Autodesk Inventor part; units mm, degrees
ref_plane "YZ Plane" through (0, 0, 0) normal (1, 0, 0) x (0, 1, 0)
ref_plane "XZ Plane" through (0, 0, 0) normal (0, 1, 0) x (-1, 0, 0)
ref_plane "XY Plane" through (0, 0, 0) normal (0, 0, 1) x (1, 0, 0)
sketch "Sketch1" plane through (0, 0, 0) normal (0, 1, 0) x (-1, 0, 0)
  line L0 (0, 0) -> (0, -62.5)
  line L1 (9.458, 0) -> (9.458, 12.5)
  line L2 (9.458, 12.5) -> (9.458, -12.5)
  line L3 (9.458, 12.5) -> (-14.404, 12.5)
  line L4 (-14.404, 12.5) -> (-14.404, -12.5)
  line L5 (-14.404, -12.5) -> (9.458, -12.5)
  line L6 (-14.404, 12.5) -> (-12.404, 12.5)
  line L7 (-14.404, -12.5) -> (-12.404, -12.5)
  circle A0 centre (0.096, 10.5) radius 1.1
  circle A1 centre (-12.404, 10.5) radius 1.1
  circle A2 centre (-12.404, -10.5) radius 1.1
  circle A3 centre (0.096, -10.5) radius 1.1
  line L8 (9.458, -62.5) -> (9.458, -50)
  line L9 (9.458, -50) -> (9.458, -75)
  line L10 (9.458, -50) -> (-14.404, -50)
  line L11 (-14.404, -50) -> (-14.404, -75)
  line L12 (-14.404, -75) -> (9.458, -75)
  line L13 (-14.404, -50) -> (-12.404, -50)
  line L14 (-14.404, -75) -> (-12.404, -75)
  circle A4 centre (0.096, -52) radius 1.1
  circle A5 centre (-12.404, -52) radius 1.1
  circle A6 centre (-12.404, -73) radius 1.1
  circle A7 centre (0.096, -73) radius 1.1
  line L15 (12.458, 15.5) -> (-17.404, 15.5)
  line L16 (-17.404, 15.5) -> (-17.404, -78)
  line L17 (-17.404, -78) -> (12.458, -78)
  line L18 (12.458, -78) -> (12.458, 15.5)
  line L19 (-14.404, -12.5) -> (-14.404, -50)
  line L20 (9.458, -50) -> (9.458, -12.5)
extrude "Extrusion1" add sketch "Sketch1" against normal blind 3 contours L5 L4 L3 L1 L2 | L5 L20 L10 L0 | L0 L10 L19 L5 | L10 L8 L9 L12 L11 | L18 L17 L16 L15
sketch "Sketch2" plane through (0, 0, 0) normal (0, 1, 0) x (1, 0, 0)
  circle A0 centre (-0.096, -10.5) radius 1.1
  circle A1 centre (-0.096, -10.5) radius 2
  circle A2 centre (12.404, -10.5) radius 1.1
  circle A3 centre (12.404, -10.5) radius 2
  circle A4 centre (12.404, 10.5) radius 1.1
  circle A5 centre (12.404, 10.5) radius 2
  circle A6 centre (-0.096, 10.5) radius 2
  circle A7 centre (-0.096, 52) radius 1.1
  circle A8 centre (-0.096, 52) radius 2
  circle A9 centre (-0.096, 73) radius 1.1
  circle A10 centre (-0.096, 73) radius 2
  circle A11 centre (12.404, 73) radius 1.1
  circle A12 centre (12.404, 73) radius 2
  circle A13 centre (12.404, 52) radius 1.1
  circle A14 centre (12.404, 52) radius 2
  circle A15 centre (-0.096, 73) radius 1.1
  circle A16 centre (12.404, 73) radius 1.1
  circle A17 centre (12.404, 52) radius 1.1
  circle A18 centre (-0.096, 52) radius 1.1
  circle A19 centre (-0.096, 10.5) radius 1.1
  circle A20 centre (12.404, 10.5) radius 1.1
  circle A21 centre (12.404, -10.5) radius 1.1
  circle A22 centre (-0.096, -10.5) radius 1.1
  circle A23 centre (-0.096, 10.5) radius 1.1
  point P0 (0, 0)
  dimension "d21" = 4
  dimension "d22" = 4
  dimension "d23" = 4
  dimension "d24" = 4
  dimension "d25" = 4
  dimension "d26" = 4
  dimension "d27" = 4
  dimension "d28" = 4
extrude "Extrusion2" add sketch "Sketch2" along normal blind 3
extrude "Extrusion3" add sketch "Sketch1" along normal blind 4 contours L18 L17 L16 L15
sketch "Sketch3" plane through (-12.458, -3, -78) normal (-1, 0, 0) x (0, 0, 1)
  line L0 (89.6, 0) -> (87.4, 0)
  line L1 (68.6, 0) -> (66.4, 0)
  line L2 (27.1, 0) -> (24.9, 0)
  line L3 (6.1, 0) -> (3.9, 0)
  line L4 (88.5, 0) -> (88.5, 3)
  line L5 (88.5, 3) -> (88.5, 5)
  line L6 (88.5, 3) -> (88.5, 6)
  line L7 (88.5, 5) -> (67.5, 5)
  line L8 (67.5, 3) -> (67.5, 6)
  line L9 (67.5, 5) -> (67.5, 3)
  line L10 (67.5, 3) -> (88.5, 3)
  line L11 (27.1, 0) -> (24.9, 0)
  line L12 (26, 0) -> (26, 5)
  line L13 (26, 5) -> (5, 5)
  line L14 (5, 3) -> (5, 6)
  line L15 (5, 5) -> (5, 3)
  line L16 (26, 3) -> (5, 3)
  line L17 (5, 3) -> (26, 3)
  dimension "d33" = 2
  dimension "d34" = 5
extrude "Extrusion4" cut sketch "Sketch3" against normal up to surface (3 mm away)
sketch "Sketch4" plane through (-12.458, -3, -78) normal (-1, 0, 0) x (0, 0, 1)
  line L0 (0, 0) -> (93.5, 0)
  line L1 (78, 0) -> (78, -30)
  line L2 (78, -30) -> (83, -30)
  line L3 (83, -30) -> (73, -30)
  line L4 (73, -30) -> (73, 0)
  line L5 (83, -30) -> (83, 0)
  line L6 (73, 0) -> (83, 0)
  line L7 (78, 3) -> (78, -30)
  point P0 (78, -30)
  point P1 (83, 0)
  point P2 (73, 0)
  dimension "d37" = 30
  dimension "d38" = 5
  dimension "d39" = 10
extrude "Extrusion5" add sketch "Sketch4" against normal up to surface (29.862 mm away)
sketch "Sketch5" plane through (-12.458, -33, 5) normal (0, 0, 1) x (1, 0, 0)
  line L0 (0, 0) -> (29.862, 0)
  line L1 (0, 30) -> (0, 0)
  circle A0 centre (14.931, 15) radius 15
  line L2 (29.862, 30) -> (29.862, 0)
  line L3 (29.862, 0) -> (29.862, 15)
  point P0 (12.458, 33)
  point P1 (29.862, 13.5629)
  point P2 (14.931, 0)
  point P3 (0, 13.5629)
extrude "Extrusion6" cut sketch "Sketch5" against normal up to surface (10 mm away) contours L1 A0 L0 | A0 L2 L0
sketch "Sketch6" plane through (-12.458, -3, 5) normal (0, 0, 1) x (1, 0, 0)
  line L0 (29.862, -30) -> (29.862, 0)
  line L1 (29.862, -16.4371) -> (26.862, -16.4371)
  circle A0 centre (26.862, -16.4371) radius 1.1
  arc A1 (0, -16.4371) -> (29.862, -16.4371) centre (14.931, -15) ccw
  circle A2 centre (14.931, -15) radius 4.093
  circle A3 centre (25.9738, -19.7402) radius 1.1
  circle A4 centre (24.191, -22.6593) radius 1.1
  circle A5 centre (21.6581, -24.9579) radius 1.1
  circle A6 centre (18.5801, -26.4498) radius 1.1
  circle A7 centre (15.2065, -27.0141) radius 1.1
  circle A8 centre (11.8106, -26.605) radius 1.1
  circle A9 centre (8.6675, -25.2558) radius 1.1
  circle A10 centre (6.0318, -23.0758) radius 1.1
  circle A11 centre (4.1171, -20.2414) radius 1.1
  circle A12 centre (3.0784, -16.9825) radius 1.1
  circle A13 centre (3, -13.5629) radius 1.1
  point P0 (12.458, 3)
  dimension "d46" = 3
  dimension "d47" = 2.2
  dimension "d50" = 180
extrude "Extrusion7" cut sketch "Sketch6" against normal up to surface (10 mm away) contours A0 | A3 | A4 | A5 | A6 | A7 | A8 | A9 | A10 | A11 | A12 | A13
sketch "Sketch7" plane through (-12.458, -3, 5) normal (0, 0, 1) x (1, 0, 0)
  arc A0 (0, -16.4371) -> (29.862, -16.4371) centre (14.931, -15) ccw
  circle A1 centre (14.931, -15) radius 2
  point P0 (12.458, 3)
  dimension "d54" = 4
extrude "Extrusion8" cut sketch "Sketch7" against normal up to surface (10 mm away)
sketch "Sketch8" plane through (0, 4, 0) normal (0, 1, 0) x (1, 0, 0)
  line L0 (17.404, -15.5) -> (17.404, 78)
  line L1 (17.404, 78) -> (-12.458, 78)
  line L2 (-12.458, 78) -> (-12.458, -15.5)
  line L3 (-12.458, -15.5) -> (17.404, -15.5)
  line L4 (14.404, 75) -> (14.404, -12.5)
  line L5 (14.404, -12.5) -> (-9.458, -12.5)
  line L6 (-9.458, -12.5) -> (-9.458, 75)
  line L7 (-9.458, 75) -> (14.404, 75)
  line L8 (-9.458, -13) -> (14.404, -13)
  line L9 (14.404, -13) -> (14.904, -13)
  line L10 (14.904, -13) -> (14.904, 75)
  line L11 (14.904, 75) -> (14.904, 75.5)
  line L12 (14.904, 75.5) -> (-9.458, 75.5)
  line L13 (-9.458, 75.5) -> (-9.958, 75.5)
  line L14 (-9.958, 75.5) -> (-9.958, -13)
  line L15 (-12.458, 78) -> (-12.458, -15.5)
  line L16 (-9.958, -13) -> (-9.458, -13)
  point P0 (0, 0)
  dimension "d57" = 0.5
  dimension "d58" = 0.5
  dimension "d59" = 0.5
  dimension "d60" = 0.5
extrude "Extrusion9" cut sketch "Sketch8" against normal up to surface (4 mm away) contours L16 L14 L13 L12 L11 L10 L9 L8
sketch "Sketch9" plane through (0, -3, 0) normal (0, -1, 0) x (1, 0, 0)
  circle A0 centre (12.404, -31.25) radius 1.45
  circle A1 centre (-0.096, -31.25) radius 1.45
  arc A2 (14.904, -29.5917) -> (14.904, -32.9083) centre (12.404, -31.25) ccw
  circle A3 centre (-0.096, -31.25) radius 3
  point P0 (0, 0)
extrude "Extrusion10" cut sketch "Sketch9" against normal up to surface (7 mm away) contours A0 | A1
sketch "Sketch10" plane through (0, -3, 0) normal (0, -1, 0) x (1, 0, 0)
  circle A0 centre (12.404, 10.5) radius 1.1
  circle A1 centre (-0.096, 10.5) radius 1.1
  circle A2 centre (12.404, -10.5) radius 1.1
  circle A3 centre (-0.096, -10.5) radius 1.1
  circle A4 centre (-0.096, -52) radius 1.1
  circle A5 centre (12.404, -52) radius 1.1
  circle A6 centre (12.404, -73) radius 1.1
  circle A7 centre (-0.096, -73) radius 1.1
  point P0 (0, 0)
extrude "Extrusion11" add sketch "Sketch10" against normal blind 3
sketch "Sketch11" plane through (0, -3, 0) normal (0, -1, 0) x (1, 0, 0)
  line L0 (17.404, -78) -> (-12.458, -78)
  line L1 (-12.458, -78) -> (-12.458, -85)
  line L2 (-12.458, -85) -> (17.404, -85)
  line L3 (17.404, -85) -> (17.404, -78)
  circle A0 centre (12.404, -81.5) radius 1.45
  circle A1 centre (0, -81.5) radius 1.45
  line L4 (-12.458, 15.5) -> (17.404, 15.5)
  line L5 (-12.458, 15.5) -> (-12.458, 22.5)
  line L6 (-12.458, 22.5) -> (17.404, 22.5)
  line L7 (17.404, 22.5) -> (17.404, 15.5)
  line L8 (17.404, 15.5) -> (-12.458, 15.5)
  line L9 (-12.458, -78) -> (17.404, -78)
  circle A2 centre (12.404, 19) radius 1.45
  circle A3 centre (0, 19) radius 1.45
  point P0 (0, 0)
  dimension "d67" = 7
  dimension "d69" = 2.9
  dimension "d70" = 2.9
  dimension "d71" = 7
  dimension "d72" = 2.9
  dimension "d73" = 2.9
extrude "Extrusion12" add sketch "Sketch11" against normal up to surface (7 mm away)
properties part number "pi_cam_stereo_board"
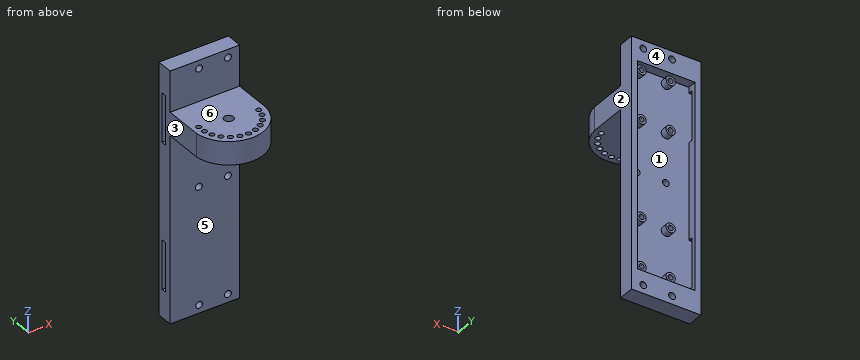
The model under review builds one solid part; all positions refer to its coordinate system, in mm. Face numbers are marked on the shaded views. A direction names the side the tool comes from. Give positions to 0.01 mm unless a question says otherwise; leave off trailing zeros. Write each loop counter-clockwise with the first axis right and the second up, starting at its lowest first coordinate (ties: lowest second). Pieces come first, ordered by that corner, then holes.
(1) The part is to be moulded in two halves that separate along X. For the marked faces 1, 2 and 3, say which applies: released by +X, released by -X, zero draft, split by the parting line, or undercut.
(2) Tool access review of the marked faces 4, 5 and 6: name each direction out of +Z, -Z, +X, -X, +Y, -Y from which nothing blocks a thin tool from reaching the whole face with its end or side.
(3) For P1, Ø2, axis at x = 14.4, y = -19.44, coming from the +Z side; P2, Ø1.5, axis at x = 7, z = -56, coming from the -Y side; P3, Ø5, axis at x = -1, y = -5, coming from the -Z side; P4, Ø4.5, axis at x = 1, z = -51, coming from the +Y side, all flat-tipped, find the tip position at first contact; note any pin that passes through.
(4) To check wall thickness, follow L1, parallel to Y at x = 14, z = 4; L2, parallel to Z at x = -3, y = -15; L3, parallel to Y at x = 3.25, z = -3. State the ranges of each line that lie inside material, in increasing order.
(5) Consider section C-C, the plane z = 19. Give the boundary of the cut face in (x, y), and give its area (3 significant figures).
(6) Consider section B-B, the plane z = -64. Give the boundary of the cut face in (x, y).
(7) Consider section A-A, the plane z = -31.25. Give the boundary of the cut face in (x, y), and give its area (3 significant figures).
Returned:
1. face 1: undercut
1. face 2: released by +X
1. face 3: released by -X
2. face 4: +Z, -Z, +X, -X, +Y
2. face 5: -Z, +X, -X, -Y
2. face 6: +Z, +X, -X, -Y
3. P1: passes through
3. P2: stops at y = -3
3. P3: stops at z = -85
3. P4: stops at y = 3
4. L1: y = -27.6 to -23.73, -21.75 to -20.46, -18.41 to 0
4. L2: z = -5 to 5
4. L3: y = -32.98 to -30.99, -29.04 to -19.84, -16.16 to 0
5. outline: (-12.46, -3) - (-1.45, -3) - (-1.45, 4) - (-12.46, 4) - close; (1.45, -3) - (10.95, -3) - (10.95, 4) - (1.45, 4) - close; (13.85, -3) - (17.4, -3) - (17.4, 4) - (13.85, 4) - close
5. area: 168 mm2
6. outline: (-12.46, -3) - (17.4, -3) - (17.4, 4) - (14.9, 4) - (14.9, 0) - (-12.46, 0) - close; (-12.46, 2) - (-9.96, 2) - (-9.96, 4) - (-12.46, 4) - close
7. outline: (-12.46, -3) - (-1.55, -3) - (-1.55, 0) - (-9.96, 0) - (-9.96, 4) - (-12.46, 4) - close; (1.35, -3) - (10.95, -3) - (10.95, 0) - (1.35, 0) - close; (13.85, -3) - (17.4, -3) - (17.4, 4) - (14.9, 4) - (14.9, 0) - (13.85, 0) - close
7. area: 92.2 mm2
